Autodesk Inventor part; units mm, degrees
ref_plane "YZ Plane" through (0, 0, 0) normal (1, 0, 0) x (0, 1, 0)
ref_plane "XZ Plane" through (0, 0, 0) normal (0, 1, 0) x (-1, 0, 0)
ref_plane "XY Plane" through (0, 0, 0) normal (0, 0, 1) x (1, 0, 0)
sketch "Эскиз1" plane through (0, 0, 0) normal (0, 1, 0) x (-1, 0, 0)
  line L0 (0, 60) -> (0, 75)
  line L1 (0, -60) -> (0, -75)
  ellipse E0 centre (0, 0) end of major axis (0, -75) minor radius 60 (60, 0) -> (0, 75) ccw
  ellipse E1 centre (0, 0) end of major axis (0, -75) minor radius 60 (-60, 0) -> (0, -75) ccw
  arc A0 (0, 60) -> (-60, 0) centre (0, 0) ccw
  arc A1 (0, -60) -> (60, 0) centre (0, 0) ccw
  circle A2 centre (0, 0) radius 30
  dimension "d1" = 75
  dimension "d2" = 75
  dimension "d5" = 60
extrude "Выдавливание1" add sketch "Эскиз1" along normal blind 350 contours L0 E0 A1 L1 E1 A0 | A2
sketch "Эскиз2" plane through (0, 0, 0) normal (0, -1, 0) x (1, 0, 0)
  ellipse E0 centre (0, 0) end of major axis (0, -75) minor radius 60 (0, 75) -> (-60, 0) ccw
  line L0 (0, 75) -> (0, 0)
  circle A0 centre (0, 0) radius 30
  line L1 (0, -75) -> (0, -60)
  line L2 (0, 0) -> (0, -75)
  line L3 (0, 0) -> (26.5165, -26.5165)
  line L4 (0, 0) -> (37.5, 0) construction
  line L5 (0, 0) -> (-26.5165, -26.5165)
  line L6 (0, 0) -> (37.5, 0) construction
  line L7 (0, 0) -> (-26.5165, 26.5165)
  line L8 (0, 0) -> (37.5, 0) construction
  line L9 (0, 0) -> (26.5165, 26.5165)
  line L10 (0, 0) -> (37.5, 0) construction
  circle A1 centre (26.5165, 26.5165) radius 5
  circle A2 centre (26.5165, -26.5165) radius 5
  circle A3 centre (-26.5165, 26.5165) radius 5
  circle A4 centre (-26.5165, -26.5165) radius 5
  circle A5 centre (0, 0) radius 45
  line L11 (0, 0) -> (30, 0)
  circle A6 centre (30, 0) radius 5
  line L12 (0, 0) -> (0, -30)
  circle A7 centre (0, -30) radius 5
  line L13 (0, 0) -> (-30, 0)
  circle A8 centre (-30, 0) radius 5
  line L14 (0, 0) -> (0, 30)
  circle A9 centre (0, 30) radius 5
  dimension "d13" = 60
  dimension "d14" = 37.5
  dimension "d15" = 45
  dimension "d16" = 37.5
  dimension "d17" = 135
  dimension "d18" = 37.5
  dimension "d19" = 135
  dimension "d20" = 37.5
  dimension "d21" = 45
  dimension "d22" = 10
  dimension "d23" = 10
  dimension "d24" = 10
  dimension "d25" = 10
  dimension "d26" = 90
  dimension "d30" = 30
  dimension "d31" = 30
  dimension "d32" = 30
  dimension "d33" = 30
hole "Отверстие1" at (0, 0, 0) direction (0, 1, 0) diameter 60 end through all counterbore diameter 90 counterbore depth 15
sketch "Эскиз3" plane through (0, 0, 0) normal (0, -1, 0) x (1, 0, 0)
  line L0 (0, 0) -> (30, 0)
  circle A0 centre (30, 0) radius 5
  line L1 (0, 0) -> (0, -30)
  circle A1 centre (0, 0) radius 30
  circle A2 centre (0, -30) radius 5
  line L2 (0, 0) -> (-30, 0)
  line L3 (0, 0) -> (0, 30)
  circle A3 centre (0, 30) radius 5
  circle A4 centre (-30, 0) radius 5
  dimension "d34" = 30
  dimension "d35" = 10
  dimension "d36" = 10
  dimension "d37" = 10
  dimension "d38" = 10
hole "Отверстие2" at (0, 0, 30) at (-30, 0, 0) at (0, 0, -30) at (30, 0, 0) direction (0, 1, 0) diameter 15 depth 45
sketch "Эскиз5" plane through (0, 350, 0) normal (0, 1, 0) x (1, 0, 0)
  circle A0 centre (0, 0) radius 45
hole "Отверстие4" at (0, 350, 0) direction (0, -1, 0) diameter 90 depth 15
sketch "Эскиз6" plane through (0, 335, 0) normal (0, 1, 0) x (1, 0, 0)
  line L0 (0, 0) -> (0, -37.5)
  line L1 (0, 0) -> (-37.5, 0)
  line L2 (0, 0) -> (0, 37.5)
  line L3 (0, 0) -> (37.5, 0)
  line L4 (0, 0) -> (-21.2132, -21.2132)
  line L5 (0, 0) -> (30, 0) construction
  line L6 (0, 0) -> (21.2132, -21.2132)
  line L7 (0, 0) -> (30, 0) construction
  line L8 (0, 0) -> (-21.2132, 21.2132)
  line L9 (0, 0) -> (30, 0) construction
  line L10 (0, 0) -> (21.2132, 21.2132)
  line L11 (0, 0) -> (30, 0) construction
  circle A0 centre (21.2132, -21.2132) radius 7.5
  circle A1 centre (-21.2132, -21.2132) radius 7.5
  circle A2 centre (-21.2132, 21.2132) radius 7.5
  circle A3 centre (21.2132, 21.2132) radius 7.5
  circle A4 centre (37.5, 0) radius 5
  circle A5 centre (0, -37.5) radius 5
  circle A6 centre (-37.5, 0) radius 5
  circle A7 centre (0, 37.5) radius 5
  dimension "d71" = 37.5
  dimension "d72" = 37.5
  dimension "d73" = 37.5
  dimension "d74" = 37.5
  dimension "d75" = 30
  dimension "d76" = 135
  dimension "d77" = 30
  dimension "d78" = 45
  dimension "d79" = 30
  dimension "d80" = 135
  dimension "d81" = 30
  dimension "d82" = 45
  dimension "d83" = 15
  dimension "d84" = 15
  dimension "d85" = 15
  dimension "d86" = 15
  dimension "d87" = 10
  dimension "d88" = 10
  dimension "d89" = 10
  dimension "d90" = 10
hole "Отверстие5" at (21.2132, 335, 21.2132) at (-21.2132, 335, 21.2132) at (-21.2132, 335, -21.2132) at (21.2132, 335, -21.2132) direction (0, -1, 0) diameter 15 depth 30
sketch "Эскиз8" plane through (0, 335, 0) normal (0, 1, 0) x (1, 0, 0)
  point P0 (37, 0)
  point P1 (0, -37)
  point P2 (-37, 0)
  point P3 (0, 37)
hole "Отверстие7" at (37, 335, 0) at (0, 335, 37) at (-37, 335, 0) at (0, 335, -37) direction (0, -1, 0) diameter 8.376 depth 8 tip angle 120
sketch "Эскиз9" plane through (0, 15, 0) normal (0, -1, 0) x (1, 0, 0)
  point P0 (26.163, 26.163)
  point P1 (26.163, -26.163)
  point P2 (-26.163, -26.163)
  point P3 (-26.163, 26.163)
hole "Отверстие8" at (26.163, 15, 26.163) at (26.163, 15, -26.163) at (-26.163, 15, -26.163) at (-26.163, 15, 26.163) direction (0, 1, 0) diameter 8.376 depth 8 tip angle 120
properties material "Сталь, литейная"
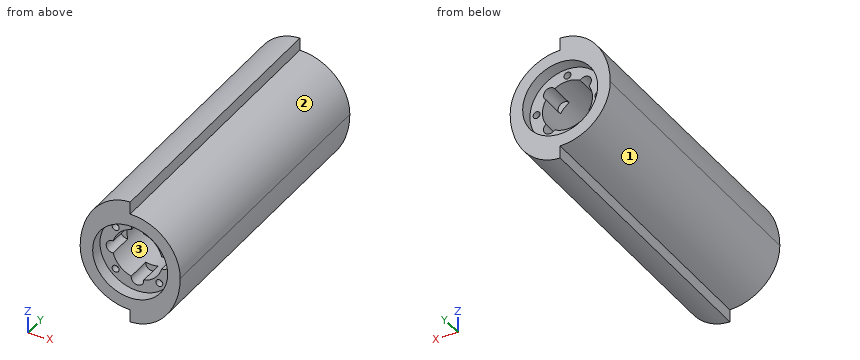
Source: CAD feature listing. Evaluate the final solid. Frame: model axes, mm. Face numbers are marked on the shaded views. Round coordinates to 2 decimals unless told otherwise and drop trailing zeros. Return JSON: item names as keys, results as strings. Group by question number.
1. Material intervals for line 1 along X through (y, z) = (162.5, 1.5); line 2 along X through (y, z) = (8, 0); line 3 along Z through (x, y) = (-17, 268.5), sorted ascending. Write a range as from..to.
2. Pin query (flat end, axial travel): pin 1 (4 mm diameter, centred on x = -22.5, z = -21.5, fed in from +Y); pin 2 (10 mm diameter, centred on x = 39.5, z = 2.5, fed in from -Y); pin 3 (15 mm diameter, centred on x = -22.5, z = 20.5, fed in from +Y). Return the tip coordinate at first contact, or that it passes through.
3. Mould query, pull axis Z, two halves, no side actions, for the marked faces 1, 2 and 3. Classes: released by +Z, released by -Z, zero draft, split by the parting line, or undercut.
Checks:
{
 "1": {"line 1": "x = -59.99..-29.96, 29.96..59.98", "line 2": "x = -60..-45, 45..60", "line 3": "z = -57.54..-24.72, 24.72..71.93"},
 "2": {"pin 1": "stops at y = 305", "pin 2": "stops at y = 15", "pin 3": "stops at y = 335"},
 "3": {"face 1": "released by -Z", "face 2": "released by +Z", "face 3": "undercut"}
}
